Autodesk Inventor part; units mm, degrees
ref_plane "YZ Plane" through (0, 0, 0) normal (1, 0, 0) x (0, 1, 0)
ref_plane "XZ Plane" through (0, 0, 0) normal (0, 1, 0) x (-1, 0, 0)
ref_plane "XY Plane" through (0, 0, 0) normal (0, 0, 1) x (1, 0, 0)
sketch "Skizze1" plane through (0, 0, 0) normal (0, 0, 1) x (1, 0, 0)
  line L0 (-7.625, -2.545) -> (2.545, -2.545)
  line L1 (2.545, -2.545) -> (2.545, 2.545)
  line L2 (2.545, 2.545) -> (1.27, 2.545)
  line L3 (1.27, 2.545) -> (1.27, 4.055)
  line L4 (1.27, 4.055) -> (-6.35, 4.055)
  line L5 (-6.35, 4.055) -> (-6.35, 2.545)
  line L6 (-6.35, 2.545) -> (-7.625, 2.545)
  line L7 (-7.625, 2.545) -> (-7.625, -2.545)
  line L8 (-5.33, 3.035) -> (0.25, 3.035)
  line L9 (0.25, 3.035) -> (0.25, 1.525)
  line L10 (0.25, 1.525) -> (1.525, 1.525)
  line L11 (1.525, 1.525) -> (1.525, -1.525)
  line L12 (1.525, -1.525) -> (-6.605, -1.525)
  line L13 (-6.605, -1.525) -> (-6.605, 1.525)
  line L14 (-6.605, 1.525) -> (-5.33, 1.525)
  line L15 (-5.33, 1.525) -> (-5.33, 3.035)
  line L16 (-6.605, 0) -> (-5.08, 0) construction
  line L17 (-5.08, 0) -> (0, 0) construction
  line L18 (0, 0) -> (1.525, 0) construction
  point P0 (0, -2.035)
  dimension "d0" = 1.02
  dimension "d1" = 3.05
  dimension "d3" = 7.62
  dimension "d4" = 6.6
  dimension "d5" = 1.525
  dimension "d6" = 5.08
extrude "Extrusion1" add sketch "Skizze1" along normal blind 3.8
sketch "Skizze2" plane through (0, 0, 0) normal (0, 0, -1) x (-1, 0, 0)
  line L0 (-2.545, -2.545) -> (-2.545, 2.545)
  line L1 (-2.545, 2.545) -> (-1.27, 2.545)
  line L2 (-1.525, 1.525) -> (-0.25, 1.525)
  line L3 (-1.525, -1.525) -> (-1.525, 1.525)
  line L4 (6.605, -1.525) -> (-1.525, -1.525)
  line L5 (7.625, -2.545) -> (-2.545, -2.545)
  line L6 (7.625, 2.545) -> (7.625, -2.545)
  line L7 (6.605, 1.525) -> (6.605, -1.525)
  line L8 (5.33, 1.525) -> (6.605, 1.525)
  line L9 (6.35, 2.545) -> (7.625, 2.545)
  line L10 (-0.25, 1.525) -> (1.04, 1.525)
  line L11 (-1.27, 2.545) -> (-1.27, 4.055)
  line L12 (-1.27, 2.545) -> (1.04, 2.545)
  line L13 (1.04, 2.545) -> (1.04, 1.525)
  line L14 (5.33, 1.525) -> (5.33, 3.035)
  line L15 (5.33, 1.525) -> (4.04, 1.525)
  line L16 (6.35, 2.545) -> (4.04, 2.545)
  line L17 (4.04, 2.545) -> (4.04, 1.525)
  point P0 (0, 0)
  dimension "d9" = 3
extrude "Extrusion2" add sketch "Skizze2" along normal blind 5.09
sketch "Skizze3" plane through (0, 0, -5.09) normal (0, 0, -1) x (-1, 0, 0)
  line L0 (-2.545, 2.545) -> (-2.545, -2.545)
  line L1 (7.625, 2.545) -> (7.625, -2.545)
  line L2 (-2.545, -2.545) -> (7.625, -2.545)
  line L3 (7.625, -2.545) -> (7.625, 2.545)
  line L4 (7.625, 2.545) -> (-2.545, 2.545)
  line L5 (-2.545, 2.545) -> (-2.545, -2.545)
  point P0 (0, 0)
extrude "Extrusion3" add sketch "Skizze3" along normal blind 2.16
sketch "Skizze4" plane through (-6.35, 4.055, 0) normal (0, 1, 0) x (1, 0, 0)
  line L0 (7.62, -3.8) -> (0, -3.8) construction
  line L1 (1.02, 0) -> (2.31, 0)
  line L2 (5.1, -2.3) -> (2.52, -2.3)
  line L3 (1.02, -0.8) -> (1.02, 0)
  line L4 (1.02, 0) -> (6.6, 0)
  line L5 (6.6, 0) -> (6.6, -0.8)
  arc A0 (5.1, -2.3) -> (6.6, -0.8) centre (5.1, -0.8) ccw
  arc A1 (1.02, -0.8) -> (2.52, -2.3) centre (2.52, -0.8) ccw
  line L6 (0, 0) -> (0, -3.8) construction
  line L7 (6.6, 0) -> (6.6, -3.8) construction
  line L8 (6.6, 0) -> (6.6, -3.8) construction
  line L9 (1.02, 0) -> (1.02, -3.8) construction
  line L10 (1.02, 0) -> (1.02, -3.8) construction
  point P0 (6.35, 0)
  dimension "d14" = 1.5
  dimension "d15" = 1.5
extrude "Extrusion4" cut sketch "Skizze4" against normal up to surface (1.02 mm away)
sketch "Skizze5" plane through (-7.625, -2.545, 3.8) normal (0, -1, 0) x (1, 0, 0)
  line L0 (0, -11.05) -> (1.2806, -11.05) construction
  line L1 (10.17, -11.05) -> (8.8894, -11.05) construction
  line L2 (1.2806, -11.05) -> (1.7194, -11.05)
  line L3 (1.7194, -11.05) -> (8.4506, -11.05) construction
  line L4 (8.4506, -11.05) -> (8.8894, -11.05)
  line L5 (8.4506, -11.05) -> (8.67, -11.43)
  line L6 (8.67, -11.43) -> (8.8894, -11.05)
  line L7 (1.7194, -11.05) -> (1.5, -11.43)
  line L8 (1.5, -11.43) -> (1.2806, -11.05)
  line L9 (10.17, -11.05) -> (10.17, 0)
  point P0 (7.625, -3.8)
  point P1 (0, -11.05)
  dimension "d18" = 0.38
  dimension "d19" = 1.5
extrude "Extrusion5" add sketch "Skizze5" against normal up to surface (5.09 mm away)
sketch "Skizze6" plane through (0, 0, -5.09) normal (0, 0, 1) x (1, 0, 0)
  line L0 (-0.32, 0.32) -> (0.32, 0.32)
  line L1 (0.32, 0.32) -> (0.32, -0.32)
  line L2 (0.32, -0.32) -> (-0.32, -0.32)
  line L3 (-0.32, -0.32) -> (-0.32, 0.32)
  line L4 (0.32, -0.32) -> (-0.32, 0.32) construction
  point P0 (0, 0)
  point P1 (0, 0)
  dimension "d22" = 0.64
extrude "Extrusion6" add sketch "Skizze6" along normal blind 6.1 and the other way blind 5.84
chamfer "Fase1" distance 0.2 angle 45 8 edges at (0, 0.32, 1.01) (0.32, 0, 1.01) (0, -0.32, 1.01) (-0.32, 0, 1.01) (0.32, 0, -10.93) (-0.32, 0, -10.93) (0, -0.32, -10.93) (0, 0.32, -10.93)
pattern_linear "Rechteckige Anordnung1" count 3 spacing 2.54 along (-1, 0, 0) of "Extrusion6", "Fase1"
sketch "Skizze8" plane through (0, 0, 3.8) normal (0, 0, 1) x (1, 0, 0)
  line L0 (1.525, -1.525) -> (-6.605, -1.525) construction
  line L1 (-7.625, -2.545) -> (2.545, -2.545) construction
  line L2 (-1.825, -2.035) -> (-3.255, -2.035) construction
  line L3 (-2.54, -2.545) -> (-2.54, -2.035) construction
  line L4 (-4.525, -1.525) -> (-3.255, -1.525)
  line L5 (-3.255, -1.525) -> (-3.255, -2.545)
  line L6 (-3.255, -2.545) -> (-4.525, -2.545)
  line L7 (-4.525, -2.545) -> (-4.525, -1.525)
  line L8 (-1.825, -1.525) -> (-0.555, -1.525)
  line L9 (-0.555, -1.525) -> (-0.555, -2.545)
  line L10 (-0.555, -2.545) -> (-1.825, -2.545)
  line L11 (-1.825, -2.545) -> (-1.825, -1.525)
  line L12 (-7.625, 2.545) -> (-7.625, -2.545)
  point P0 (0, 0)
  dimension "d33" = 1.27
  dimension "d34" = 3.1
extrude "Extrusion7" cut sketch "Skizze8" against normal up to surface (8.89 mm away) contours L8 L9 L10 L11
chamfer "Fase2" distance 0.51 angle 45 9 edges at (-6.605, 0, 3.8) (-4.215, -1.525, 3.8) (-5.9675, 1.525, 3.8) (-5.33, 2.28, 3.8) (-2.54, 3.035, 3.8) (0.25, 2.28, 3.8) (0.8875, 1.525, 3.8) (1.525, 0, 3.8) (0.485, -1.525, 3.8)
properties part number "Molex_3"
Here's how the part is built. I have some questions about the finished solid (model axes, mm). A direction names the side the tool comes from. Coordinates: 2 decimals unless noted, no trailing zeros. Loops run counter-clockwise (first coordinate to the right, second up) from the corner with the lowest first, then second, coordinate; pieces in that order, holes last. Notation, with made-up numbers: M -8,51.25 L 35,51.25 A19 ccw 35,80.25 Z; hole C 22.5,29.5 d7. An arc over 180 degrees is marked long. One line per item, written item: value.
1. Imagine slicing it at D-D (z = -9.5). List the corners of the cut face in (x, y) for me, and give its area (3 significant figures).
Geometry says:
outline: M -5.4,-0.32 L -4.76,-0.32 L -4.76,0.32 L -5.4,0.32 Z; M -2.86,-0.32 L -2.22,-0.32 L -2.22,0.32 L -2.86,0.32 Z; M -0.32,-0.32 L 0.32,-0.32 L 0.32,0.32 L -0.32,0.32 Z
area: 1.23 mm2
2. Thinking about a two-plate mould opening in Y: for faces 5 (the flat face through (-2, -2.545, -2)), 6 (the flat face through (-5.33, 2, 1)), 7 (the flat face through (-1.04, 2, -3)), which applies, +Y half, -Y half, draft (parallel to the pull), parting line (faces both ways), or undercut?
Geometry says:
face 5: -Y half
face 6: undercut
face 7: draft
3. Please list where these lines run through material, in increasing order: probe 1 along X at (y, z) = (0, -2.25) (3 decimals); probe 2 along Y at (x, z) = (0.25, -0.25) (3 decimals); probe 3 along X at (y, z) = (2.5, 2.5) (3 decimals).
Geometry says:
probe 1: x = -7.625 to -6.605, -5.4 to -4.76, -2.86 to -2.22, -0.32 to 0.32, 1.525 to 2.545
probe 2: y = -2.545 to -1.525, -0.32 to 0.32, 1.525 to 2.545
probe 3: x = -7.625 to -5.33, 0.25 to 2.545
4. Imagine slicing it at C-C (y = 2.75). List the corners of the cut face in (x, z) for me, and give its area (3 significant figures).
Geometry says:
outline: M -6.35,0 L -5.33,0 L -5.33,3.29 L -5.84,3.8 L -6.35,3.8 Z; M 0.25,0 L 1.27,0 L 1.27,3.8 L 0.76,3.8 L 0.25,3.29 Z
area: 7.49 mm2
5. Imagine slicing it at A-A (z = 0.5). State how many separate pieces and enclosed holes the cut face has, and give its area (3 significant figures).
Geometry says:
separate pieces: 5
enclosed holes: 0
area: 24.3 mm2
6. Will these pins go through, and if not, where does the flat tip stop? pin 1 Ø4 at (x, z) = (-2, -3) entering from +Y (3 decimals); pin 2 Ø2 at (x, y) = (0, 1.5) entering from +Z; pin 3 Ø1.1 at (x, y) = (1, 3.5) entering from -Z; pin 4 Ø0.8 at (x, y) = (-5, 2) entering from +Z.
Geometry says:
pin 1: stops at y = 2.545
pin 2: stops at z = 3.8
pin 3: stops at z = 0
pin 4: stops at z = 3.36
7. Imagine slicing it at B-B (x = -1.5). List the corners of the cut face in (y, z) for me (3 decimals), and give its area (3 significant figures).
Geometry says:
outline: M -2.545,-7.25 L 2.545,-7.25 L 2.545,-5.09 L -2.545,-5.09 Z; M 3.035,2.3 L 4.055,2.3 L 4.055,3.8 L 3.545,3.8 L 3.035,3.29 Z
area: 12.4 mm2
8. On a 3-axis mill with a long thin cutter (end or side, diameter ignored), from which of +Z, -Z, +X, -X, +Y, -Y can I reach the whole of each face in a straight line? I mean faces 1 (the flat face through (1, 3, 0)), 2 (the cylindrical face through (-0.2, 3.55, 1.87)), 3 (the flat face through (1.27, 3, 2)), 4 (the flat face through (-4, -1.525, -1)). Say none if no direction works.
Geometry says:
face 1: -Z, +X, -X, +Y
face 2: -Z, +Y
face 3: +Z, -Z, +X, +Y
face 4: +Z
